Model file for the job. Use its own axes, mm. Give positions to 0.01 mm unless a question says otherwise; leave off trailing zeros. Write each loop counter-clockwise with the first axis right and the second up, starting at its lowest first coordinate (ties: lowest second). Pieces come first, ordered by that corner, then holes. Notation, with made-up numbers: (-2, 77.5) - (10, 77.5) arc R11 ccw to (10, 98.5) - close; hole circle Ø2 at (82, 10). An arc over 180 degrees is marked (long way). Use CSV: the item, a comma, the result in double quotes.
from build123d import *

# Parameters (mm, degrees)
TD_SKETCH_R                   = 0.79248
TL_FEATURE_DEPTH              = 21.0312
TDF_STD_SKETCH_W              = 1.60495996
TDF_STD_SKETCH_H              = 1.60495996
TDF_STD_FEATURE_DEPTH         = 22.061040395
ISA_20_STD_FEATURE_DEPTH      = 22.061040395
ISA_20_STD_FEATURE_DEPTH_BACK = 22.061040395
F_10BA_STD_FEATURE_DEPTH      = 22.061040395
F_10BA_STD_FEATURE_DEPTH_BACK = 22.061040395


with BuildPart() as part:
    # TD_sketch → TL_feature (new body)
    with BuildSketch(Plane(origin=(0, 0, 0), x_dir=(1, 0, 0), z_dir=(0, 1, 0))):
        with Locations(Location((0, 0, 0), (0, 0, 270))):
            Circle(TD_SKETCH_R)
    extrude(amount=TL_FEATURE_DEPTH)

    # TDF_STD_sketch → TDF_STD_feature (cut, through all)
    with BuildSketch(Plane(origin=(0, 0, 0), x_dir=(1, 0, 0), z_dir=(0, 1, 0))):
        with Locations((-1.17839998, 0)):
            Rectangle(TDF_STD_SKETCH_W, TDF_STD_SKETCH_H)
    extrude(amount=TDF_STD_FEATURE_DEPTH, mode=Mode.SUBTRACT)

    # ISA_20_STD_sketch → ISA_20_STD_feature (cut, two sides: drawn at the far end of the back side and taken through both)
    with BuildSketch(Plane(origin=(0, 0, 0), x_dir=(0, 0, -1), z_dir=(1, 0, 0)).offset(-ISA_20_STD_FEATURE_DEPTH_BACK)):
        Polygon((-12.996080373, 73.27228267), (-3.784567997, 21.0312), (-0.0762, 0), (0.0762, 0), (3.784567997, 21.0312), (12.996080373, 73.27228267), (12.996080373, -32.821688483), (-12.996080373, -32.821688483), align=None)
    extrude(amount=ISA_20_STD_FEATURE_DEPTH + ISA_20_STD_FEATURE_DEPTH_BACK, mode=Mode.SUBTRACT)

    # 10BA_STD_sketch → 10BA_STD_feature (cut, two sides: drawn at the far end of the back side and taken through both)
    with BuildSketch(Plane.XY.offset(-F_10BA_STD_FEATURE_DEPTH_BACK)):
        Polygon((-53.216424634, 0), (-0.37592, 0), (-0.29972, 0), (-0.011354365, 0.050846642), (3.688047997, 21.0312), (12.863705333, 73.068938636), (91.245889802, 2.18375769), (25.165759835, -70.885180946), align=None)
    extrude(amount=F_10BA_STD_FEATURE_DEPTH + F_10BA_STD_FEATURE_DEPTH_BACK, mode=Mode.SUBTRACT)


solid = part.part
(1) Saw through at B-B, the plane z = -0.3. List the corners of the cut face in (x, y).
Checked values:
outline,"(-0.38, 1.27) - (0.2, 1.27) - (0.73, 4.28) - (0.73, 21.03) - (-0.38, 21.03) - close"
(2) Saw through at C-C, the plane x = 0.3. List the corners of the cut face in (y, z), then the cut area to 3 significant figures.
Checked values:
outline,"(1.82, -0.4) - (3.73, -0.73) - (21.03, -0.73) - (21.03, 0.73) - (3.73, 0.73) - (1.82, 0.4) - close"
area,"27.5 mm^2"
(3) Wall check: probe 1 along X at (y, z) = (13, 0.05); probe 2 along X at (y, z) = (19.75, 0.3); probe 3 along Z at (x, y) = (-0.25, 1). Give the ranges that are in metal, low to high. Write a range as [from, to].
Checked values:
probe 1,"x = [-0.38, 0.79]"
probe 2,"x = [-0.38, 0.73]"
probe 3,"z = [-0.25, 0.25]"
(4) Saw through at A-A, the plane y = 5.75. List the corners of the cut face in (x, z).
Checked values:
outline,"(-0.38, -0.7) arc R0.79 ccw (long way) to (-0.38, 0.7) - close"
